from build123d import *

# Parameters (mm, degrees)
SKETCH1_W           = 50.8
SKETCH1_H           = 50.8
BOSS_EXTRUDE1_DEPTH = 4.7625
CUT_EXTRUDE1_REACH  = 38.235
SKETCH2_R           = 12.7


with BuildPart() as part:
    # Sketch1 → Boss-Extrude1 (new body)
    with BuildSketch(Plane(origin=(0, 0, 0), x_dir=(1, 0, 0), z_dir=(0, 1, 0))):
        Rectangle(SKETCH1_W, SKETCH1_H)
    extrude(amount=BOSS_EXTRUDE1_DEPTH)

    # Sketch2 → Cut-Extrude1 (cut, up to next)
    with BuildSketch(Plane(origin=(0, 4.7625, 0), x_dir=(1, 0, 0), z_dir=(0, 1, 0)), mode=Mode.PRIVATE) as cut_extrude1_sk1:
        with Locations(Location((0, 0, 0), (0, 0, 270))):
            Circle(SKETCH2_R)
    cut_extrude1_tool1 = extrude(cut_extrude1_sk1.sketch, amount=-CUT_EXTRUDE1_REACH, mode=Mode.PRIVATE) & part.part
    add(cut_extrude1_tool1.solids().sort_by_distance((0, 4.7625, 0))[0], mode=Mode.SUBTRACT)


solid = part.part
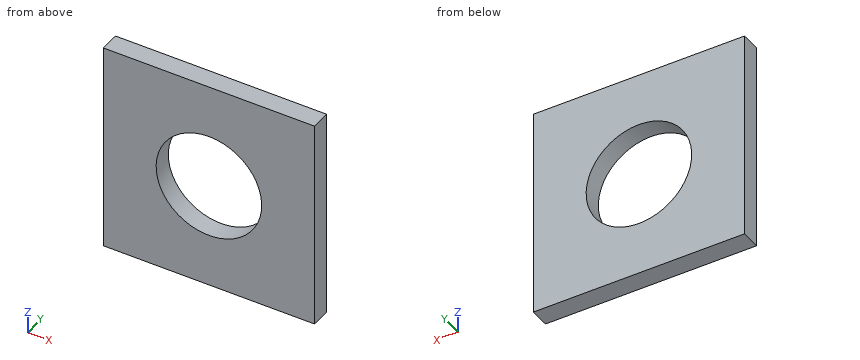
Input: part model. Units: mm. Frame: model coordinates. Round coordinates to 2 decimals unless told otherwise and drop trailing zeros. Loops run counter-clockwise (first coordinate to the right, second up) from the corner with the lowest first, then second, coordinate; pieces in that order, holes last. Notation, with made-up numbers: (6, -19.5) -> (25, -19.5) arc R12 cw to (25, -11.5) -> close; hole circle Ø8 at (64.5, -5). An arc over 180 degrees is marked (long way). Answer as a JSON object with one key per item and string values. Group by question number.
1) Ray query, L1, parallel to X at y = 2.9, z = 0; L2, parallel to Z at x = 3.5, y = 0.75; L3, parallel to X at y = 3.3, z = -2.5. Return the intervals inside material, ascending.
2) Section query A-A on x = 0. Output: boundary loops of the cut face in (y, z).
3) Section query C-C on y = 1.4. Output: boundary loops of the cut face in (x, z), plus the area to 3 significant figures.
4) Section query B-B on z = 0. Output: boundary loops of the cut face in (x, y), plus the area to 3 significant figures.
Reply:
{
 "1": {"L1": "x = -25.4 to -12.7, 12.7 to 25.4", "L2": "z = -25.4 to -12.21, 12.21 to 25.4", "L3": "x = -25.4 to -12.45, 12.45 to 25.4"},
 "2": {"outline": "(0, -25.4) -> (4.76, -25.4) -> (4.76, -12.7) -> (0, -12.7) -> close; (0, 12.7) -> (4.76, 12.7) -> (4.76, 25.4) -> (0, 25.4) -> close"},
 "3": {"outline": "(-25.4, -25.4) -> (25.4, -25.4) -> (25.4, 25.4) -> (-25.4, 25.4) -> close; hole circle Ø25.4 at (0, 0)", "area": "2,070 mm2"},
 "4": {"outline": "(-25.4, 0) -> (-12.7, 0) -> (-12.7, 4.76) -> (-25.4, 4.76) -> close; (12.7, 0) -> (25.4, 0) -> (25.4, 4.76) -> (12.7, 4.76) -> close", "area": "121 mm2"}
}
